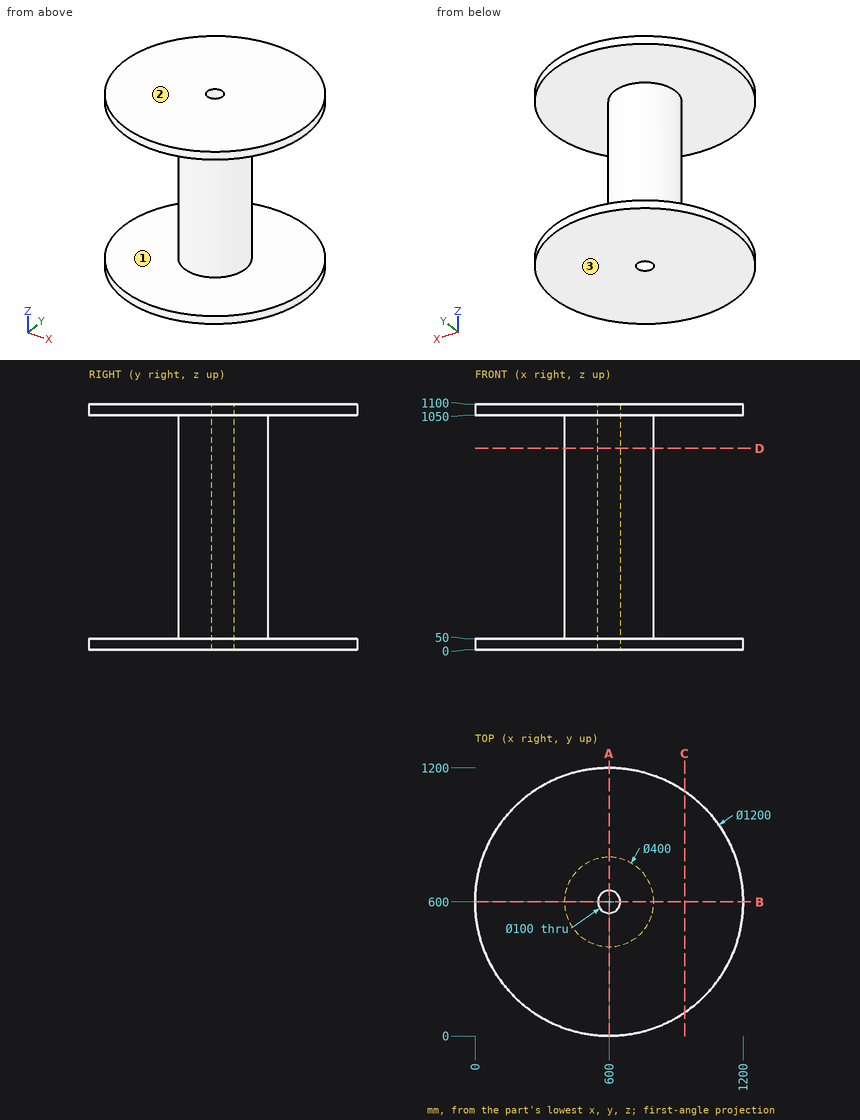
Input: dimensioned drawing with shaded views. Units: mm. Origin: part minimum x, y, z. Coordinates: 2 decimals unless noted, no trailing zeros. Write each loop counter-clockwise with the first axis right and the second up, starting at its lowest first coordinate (ties: lowest second). Pieces come first, ordered by that corner, then holes. Notation, with made-up numbers: M -8,-9.75 L 0,-9.75 A13 ccw 0,9.25 Z; hole C 85.25,74 d9. An arc over 180 degrees is marked long. Use one line per item in the form item = value.
Q1. Material intervals for probe 1 along Z at (x, y) = (1023, 406); probe 2 along Y at (x, z) = (600, 300); probe 3 along X at (y, z) = (616, 639), sorted ascending. Write a range as from..to.
Answer below:
probe_1 = 0..50, 1050..1100
probe_2 = 400..550, 650..800
probe_3 = 400.64..552.63, 647.37..799.36
Q2. First-contact query: pin 1 (1 mm diameter, centred on y = 680.5, z = 775, fed in from +X). Flat tip, straight axial feed; report the tip coordinate or a pass-through.
Answer below:
pin_1 = 783.3
Q3. Section C-C (x = 938.5). Return loops of the section in (y, z), plus the area to 3 significant figures.
Answer below:
outline = M 104.6,0 L 1095.4,0 L 1095.4,50 L 104.6,50 Z; M 104.6,1050 L 1095.4,1050 L 1095.4,1100 L 104.6,1100 Z
area = 99,100 mm²
Q4. Draft query along Z for the marked faces 1, 2 and 3. Return one class per face: released by +Z, released by -Z, zero draft, split by the parting line, or undercut.
Answer below:
face_1 = undercut
face_2 = released by +Z
face_3 = released by -Z
Q5. Section D-D (z = 901). Return loops of the section in (x, y).
Answer below:
outline = C 600,600 d400; hole C 600,600 d100
Q6. Section A-A (x = 600). Return loops of the section in (y, z), plus the area to 3 significant figures.
Answer below:
outline = M 0,0 L 550,0 L 550,1100 L 0,1100 L 0,1050 L 400,1050 L 400,50 L 0,50 Z; M 650,0 L 1200,0 L 1200,50 L 800,50 L 800,1050 L 1200,1050 L 1200,1100 L 650,1100 Z
area = 410,000 mm²
